Build history of the part. All positions in model axes, mm. Round coordinates to 2 decimals unless told otherwise and drop trailing zeros. Write each loop counter-clockwise with the first axis right and the second up, starting at its lowest first coordinate (ties: lowest second). Pieces come first, ordered by that corner, then holes. Notation, with made-up numbers: (62, -25) -> (93, -25) arc R18 cw to (93, -12) -> close; hole circle Ø5 at (14, -4). An arc over 180 degrees is marked (long way). Answer in a Markdown table with one row per item. Add a question column.
Autodesk Inventor part; units mm, degrees
ref_plane "YZ Plane" through (0, 0, 0) normal (1, 0, 0) x (0, 1, 0)
ref_plane "XZ Plane" through (0, 0, 0) normal (0, 1, 0) x (-1, 0, 0)
ref_plane "XY Plane" through (0, 0, 0) normal (0, 0, 1) x (1, 0, 0)
sketch "Esboço1" plane through (0, 0, 0) normal (0, 1, 0) x (-1, 0, 0)
  line L0 (0, 0) -> (150, 0)
  line L1 (150, 0) -> (150, -150)
  line L2 (150, -150) -> (0, -150)
  line L3 (0, -150) -> (0, 0)
  dimension "d0" = 150
  dimension "d1" = 150
extrude "Extrusão1" add sketch "Esboço1" along normal blind 8
sketch "Esboço2" plane through (0, 8, 0) normal (0, 1, 0) x (1, 0, 0)
  line L0 (-135, 15) -> (-15, 15)
  line L1 (-15, 15) -> (-15, 135)
  line L2 (-15, 135) -> (-135, 135)
  line L3 (-135, 135) -> (-135, 15)
  line L4 (0, 150) -> (-150, 150)
  line L5 (0, 0) -> (0, 150)
  point P0 (-75, 135)
  point P1 (-75, 150)
  point P2 (0, 75)
  point P3 (-135, 75)
  dimension "d4" = 120
  dimension "d5" = 120
  dimension "d6" = 0
  dimension "d7" = 0
extrude "Extrusão2" cut sketch "Esboço2" against normal blind 5
sketch "Esboço3" plane through (0, 3, 0) normal (0, 1, 0) x (1, 0, 0)
  line L0 (-120, 20) -> (-30, 20)
  line L1 (-20, 30) -> (-20, 120)
  line L2 (-30, 130) -> (-120, 130)
  line L3 (-130, 120) -> (-130, 30)
  line L4 (-135, 15) -> (-135, 135)
  line L5 (-135, 135) -> (-15, 135)
  arc A0 (-120, 130) -> (-130, 120) centre (-120, 120) ccw
  arc A1 (-20, 120) -> (-30, 130) centre (-30, 120) ccw
  arc A2 (-30, 20) -> (-20, 30) centre (-30, 30) ccw
  arc A3 (-130, 30) -> (-120, 20) centre (-120, 30) ccw
  point P0 (0, 0)
  point P1 (-130, 20)
  point P2 (-20, 130)
  point P3 (-20, 20)
  point P4 (-130, 130)
  point P5 (-135, 75)
  point P6 (-130, 75)
  point P7 (-75, 135)
  point P8 (-75, 130)
  dimension "d10" = 110
  dimension "d11" = 0
  dimension "d12" = 0
  dimension "d52" = 10
extrude "Extrusão3" cut sketch "Esboço3" against normal up to surface (3 mm away)
sketch "Esboço4" plane through (0, 8, 0) normal (0, 1, 0) x (1, 0, 0)
  circle A0 centre (-15, 15) radius 5
  circle A1 centre (-135, 15) radius 5
  circle A2 centre (-135, 135) radius 5
  circle A3 centre (-15, 135) radius 5
  line L0 (-15, 135) -> (-15, 15)
  line L1 (-15, 15) -> (-135, 15)
  line L2 (-135, 15) -> (-135, 135)
  line L3 (-135, 135) -> (-15, 135)
  point P0 (0, 0)
  dimension "d15" = 10
  dimension "d16" = 0
  dimension "d17" = 0
  dimension "d18" = 0
  dimension "d19" = 0
  dimension "d20" = 0
  dimension "d21" = 0
  dimension "d22" = 0
  dimension "d23" = 0
extrude "Extrusão4" cut sketch "Esboço4" against normal blind 5 contours A0 L1 L0 | L0 L1 A0 | L0 L3 A3 | A3 L3 L0 | L1 L2 A1 | A1 L2 L1 | L3 L2 A2 | A2 L2 L3
sketch "Esboço5" plane through (-150, 0, 0) normal (0, 0, 1) x (1, 0, 0)
  line L0 (130, 3) -> (20, 3)
  line L1 (0, 8) -> (150, 8)
  point P0 (150, 0)
  point P1 (75, 5.5)
  point P2 (75, 8)
  dimension "d26" = 5
  dimension "d27" = 2.5
  dimension "d28" = 0
hole "Furo1" at (-75, 5.5, 0) direction (0, 0, -1) diameter 2.459 end up to surface
sketch "Esboço6" plane through (0, 8, 0) normal (0, 1, 0) x (1, 0, 0)
  line L0 (-150, 150) -> (-150, 0)
  line L1 (-135, 20) -> (-135, 130)
  line L2 (0, 150) -> (-150, 150)
  line L3 (0, 0) -> (0, 150)
  line L4 (-150, 0) -> (0, 0)
  point P0 (-142.5, 7.5)
  point P1 (-142.5, 142.5)
  point P2 (-7.5, 142.5)
  point P3 (-7.5, 7.5)
  point P4 (-135, 75)
  point P5 (-150, 75)
  dimension "d36" = 7.5
  dimension "d37" = 15
  dimension "d38" = 7.5
  dimension "d39" = 7.5
  dimension "d40" = 7.5
  dimension "d41" = 7.5
  dimension "d42" = 7.5
  dimension "d43" = 7.5
  dimension "d44" = 7.5
hole "Furo2" at (-142.5, 8, -7.5) at (-142.5, 8, -142.5) at (-7.5, 8, -142.5) at (-7.5, 8, -7.5) direction (0, -1, 0) diameter 5 depth 8 counterbore diameter 8.5 counterbore depth 5
chamfer "Chamfer1" distance 0.5 angle 45 8 edges at (-150, 8, -75) (-75, 8, -150) (0, 8, -75) (-75, 8, 0) (-75, 8, -15) (-15, 8, -75) (-75, 8, -135) (-135, 8, -75)
equation "\"Raio_vergadura\" = Espessura"
equation "\"Largura_alívio_de_vergadura\" = Espessura"
equation "\"Profundidade_alívio_de_vergadura\" = 0.5 * Espessura"
equation "\"Tamanho_alívio_de_dobra\" = 4 * Espessura"
equation "\"Remanescente_mínimo\" = 2 * Espessura"
equation "\"Raiodetransição\" = Raio_vergadura"
equation "\"Tamanho_de_raio_de_Jacobi\" = Raio_vergadura"
equation "\"TamanhoFolga\" = Espessura"
properties part number "Suporte base da mesa" material "Brass, Soft Yellow"
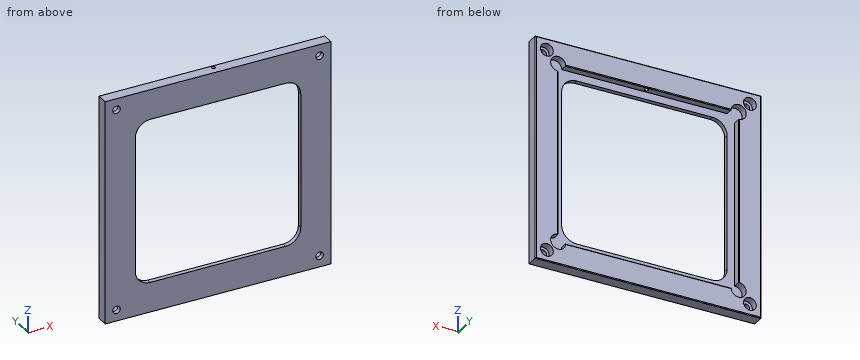
(1) Saw through at A-A (z = -97). List the corners of the cut face in (x, y), plus the area to 4 significant figures.
(2) Saw through at C-C (x = -142.5). List the corners of the cut face in (y, z).
(3) Probe line 1 along X through (y, z) = (3.75, -142); line 2 along Z through (x, y) = (-142.5, 5.4); line 3 along Z through (x, y) = (-63.5, 7.25). List the from-to ranges inside material, lowest first.
(4) Saw through at B-B (x = -70). List the corners of the cut face in (y, z).
(5) Drop a flat-ended pin along its axis: P1, Ø6.5, axis at x = -142.5, z = -7.5, coming from the +Y side. Give the stop position or say it passes through.
Answer sheet:
| question | item | result |
|---|---|---|
| 1 | outline | (-150, 0) -> (-130, 0) -> (-130, 3) -> (-135, 3) -> (-135, 7.5) -> (-135.5, 8) -> (-149.5, 8) -> (-150, 7.5) -> close; (-20, 0) -> (0, 0) -> (0, 7.5) -> (-0.5, 8) -> (-14.5, 8) -> (-15, 7.5) -> (-15, 3) -> (-20, 3) -> close |
| 1 | area | 269.5 mm² |
| 2 | outline | (0, -150) -> (7.5, -150) -> (8, -149.5) -> (8, -146.75) -> (3, -146.75) -> (3, -145) -> (0, -145) -> close; (0, -140) -> (3, -140) -> (3, -138.25) -> (8, -138.25) -> (8, -11.75) -> (3, -11.75) -> (3, -10) -> (0, -10) -> close; (0, -5) -> (3, -5) -> (3, -3.25) -> (8, -3.25) -> (8, -0.5) -> (7.5, 0) -> (0, 0) -> close |
| 3 | line 1 | x = -150 to -146.72, -138.28 to -11.72, -3.28 to 0 |
| 3 | line 2 | z = -150 to -146.75, -138.25 to -11.75, -3.25 to 0 |
| 3 | line 3 | z = -150 to -135, -15 to 0 |
| 4 | outline | (0, -150) -> (7.5, -150) -> (8, -149.5) -> (8, -135.5) -> (7.5, -135) -> (3, -135) -> (3, -130) -> (0, -130) -> close; (0, -20) -> (3, -20) -> (3, -15) -> (7.5, -15) -> (8, -14.5) -> (8, -0.5) -> (7.5, 0) -> (0, 0) -> close |
| 5 | P1 | stops at y = 3 |
